```python
from build123d import *

# Parameters (mm, degrees)
SM_BASE_FLANGE_1_DEPTH = 12
SKETCH_2_R             = 25
CUT_EXTRUDE_1_DEPTH    = 184.967388414
FILLET_1_R             = 3


# Sheet-metal steps are written as plain solids
with BuildPart() as part:
    # Sketch 1 → 基体-法兰1 (new body)
    with BuildSketch(Plane.XY):
        with BuildLine():
            Line((-30, 0), (-90, -80))
            Line((-90, -80), (-90, -150))
            ThreePointArc((-90, -150), (-87.071067812, -157.071067812), (-80, -160))
            Line((-80, -160), (0, -160))
            Line((0, -160), (0, 0))
            Line((0, 0), (-30, 0))
        make_face()
    extrude(amount=-SM_BASE_FLANGE_1_DEPTH)

    # Sketch 2 → 切除-拉伸1 (cut, through all)
    with BuildSketch(Plane.XY):
        with Locations((-40, -100)):
            Circle(SKETCH_2_R)
    extrude(amount=-CUT_EXTRUDE_1_DEPTH, mode=Mode.SUBTRACT)

    # 圆角1
    fillet_1_edges = [part.edges().sort_by_distance(p)[0] for p in [
        (-65, -100, -12),
        (-65, -100, 0),
    ]]
    fillet(fillet_1_edges, radius=FILLET_1_R)


solid = part.part
```
CAD build for the part. Positions are in the model's coordinates, mm. Round coordinates to 2 decimals unless told otherwise and drop trailing zeros. Write each loop counter-clockwise with the first axis right and the second up, starting at its lowest first coordinate (ties: lowest second). Pieces come first, ordered by that corner, then holes. Notation, with made-up numbers: (-24, -18) - (19, -18) arc R32 ccw to (19, 15) - close; hole circle Ø5 at (-4.75, -18). An arc over 180 degrees is marked (long way). Return JSON: item names as keys, results as strings. Group by question number.
Item 1: Probe probe 1 along Y at (x, z) = (-40, -5.8); probe 2 along X at (y, z) = (-107, -6.25); probe 3 along X at (y, z) = (-86, -2.25). List the from-to ranges inside material, lowest first.
Item 2: Flat gauge pin, fed straight in: pin 1 Ø5 at (y, z) = (-16, -7.5) entering from -X (3 decimals). Where does the tip first touch, or does it go through?
Item 3: Band-saw the part on C-C on y = -49. List the corners of the cut face in (x, z).
Item 4: Band-saw the part on D-D on y = -15.5. List the corners of the cut face in (x, z) (3 decimals).
Item 5: Mould opens along X. For faces 1 (the face through (-15, 0, -6)), 2 (the face through (-60, -115, -6)), 3 (the face through (0, -81, -6)), 4 (the face through (-90, -115, -6)) say: +X half, -X half, draft (parallel to the pull), parting line (faces both ways), or undercut.
Item 6: Band-saw the part on A-A on y = -100. List the corners of the cut face in (x, z), plus the area to 3 significant figures.
Item 7: Band-saw the part on B-B on x = -40. List the corners of the cut face in (y, z).
Resolved:
{
 "1": {"probe 1": "y = -160 to -125, -75 to -13.33", "probe 2": "x = -90 to -64, -16 to 0", "probe 3": "x = -90 to -60.83, -19.17 to 0"},
 "2": {"pin 1": "stops at x = -43.875"},
 "3": {"outline": "(-66.75, -12) - (0, -12) - (0, 0) - (-66.75, 0) - close"},
 "4": {"outline": "(-41.625, -12) - (0, -12) - (0, 0) - (-41.625, 0) - close"},
 "5": {"face 1": "draft", "face 2": "undercut", "face 3": "+X half", "face 4": "-X half"},
 "6": {"outline": "(-90, -12) - (-68, -12) arc R3 ccw to (-65, -9) - (-65, -3) arc R3 ccw to (-68, 0) - (-90, 0) - close; (-15, -9) arc R3 ccw to (-12, -12) - (0, -12) - (0, 0) - (-12, 0) arc R3 ccw to (-15, -3) - close", "area": "472 mm²"},
 "7": {"outline": "(-160, -12) - (-128, -12) arc R3 ccw to (-125, -9) - (-125, -3) arc R3 ccw to (-128, 0) - (-160, 0) - close; (-75, -9) arc R3 ccw to (-72, -12) - (-13.33, -12) - (-13.33, 0) - (-72, 0) arc R3 ccw to (-75, -3) - close"}
}
